Here's how the part is built. I have some questions about the finished solid (model axes, mm). Face numbers are marked on the shaded views. A direction names the side the tool comes from. Round coordinates to 2 decimals unless told otherwise and drop trailing zeros. Order: outer loops, then holes, each group sorted by start corner. A loop starts at its lowest first (then second) coordinate and runs counter-clockwise, first axis right, second up. Notation, with made-up numbers: (64.25, 53.5) -> (75.25, 53.5) arc R37 cw to (75.25, 90.5) -> close; hole circle Ø8 at (88, 12). An arc over 180 degrees is marked (long way). Use a Markdown table: item, result. Add a question column.
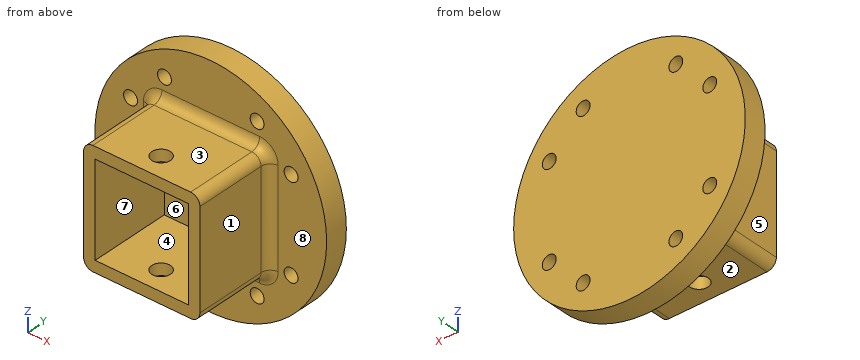
from build123d import *

# Parameters (mm, degrees)
SKETCH2_R               = 31.75
BOSS_EXTRUDE1_DEPTH     = 6.35
SKETCH3_W               = 31.877
SKETCH3_H               = 31.877
BOSS_EXTRUDE2_DEPTH     = 22.225
SKETCH4_W               = 25.527
SKETCH4_H               = 25.527
CUT_EXTRUDE1_DEPTH      = 23.225
SKETCH5_R               = 1.90000001
CUT_EXTRUDE2_DEPTH      = 7.35
SKETCH7_R               = 2.563499953
CUT_EXTRUDE3_DEPTH      = 32.75
CUT_EXTRUDE3_DEPTH_BACK = 32.75
CIRPATTERN2_COUNT       = 4
FILLET2_R               = 2.54
FILLET3_R               = 2.54


with BuildPart() as part:
    # Sketch2 → Boss-Extrude1 (new body)
    with BuildSketch(Plane(origin=(0, 0, 0), x_dir=(1, 0, 0), z_dir=(0, 1, 0))):
        Circle(SKETCH2_R)
    extrude(amount=BOSS_EXTRUDE1_DEPTH)

    # Sketch3 → Boss-Extrude2 (add)
    with BuildSketch(Plane(origin=(0, 0, 0), x_dir=(1, 0, 0), z_dir=(0, 1, 0))):
        Rectangle(SKETCH3_W, SKETCH3_H)
    extrude(amount=-BOSS_EXTRUDE2_DEPTH)

    # Sketch4 → Cut-Extrude1 (cut, through all)
    with BuildSketch(Plane(origin=(0, 0, 0), x_dir=(1, 0, 0), z_dir=(0, 1, 0))):
        Rectangle(SKETCH4_W, SKETCH4_H)
    extrude(amount=-CUT_EXTRUDE1_DEPTH, mode=Mode.SUBTRACT)

    # Sketch5 → Cut-Extrude2 (cut, through all)
    with BuildSketch(Plane(origin=(0, 0, 0), x_dir=(1, 0, 0), z_dir=(0, 1, 0))):
        with Locations((21.997045256, 12.7)):
            Circle(SKETCH5_R)
        with Locations((21.997045256, -12.7)):
            Circle(SKETCH5_R)
    cut_extrude2 = extrude(amount=CUT_EXTRUDE2_DEPTH, mode=Mode.SUBTRACT)

    # Sketch7 → Cut-Extrude3 (cut, two sides)
    with BuildSketch(Plane.XY) as cut_extrude3_sk:
        with Locations((0, -16.002)):
            Circle(SKETCH7_R)
    extrude(amount=CUT_EXTRUDE3_DEPTH, mode=Mode.SUBTRACT)
    extrude(cut_extrude3_sk.sketch, amount=-CUT_EXTRUDE3_DEPTH_BACK, mode=Mode.SUBTRACT)

    # CirPattern2: Cut-Extrude2 ×4 about axis
    cirpattern2_axis = Axis((0, 0, 0), (0, 1, 0))
    for i in range(1, CIRPATTERN2_COUNT):
        add(cut_extrude2.rotate(cirpattern2_axis, i * 360 / CIRPATTERN2_COUNT), mode=Mode.SUBTRACT)

    # Fillet2
    fillet2_edges = [part.edges().sort_by_distance(p)[0] for p in [
        (-15.9385, -11.1125, -15.9385),
        (15.9385, -11.1125, -15.9385),
        (15.9385, -11.1125, 15.9385),
        (-15.9385, -11.1125, 15.9385),
    ]]
    fillet(fillet2_edges, radius=FILLET2_R)

    # Fillet3
    fillet3_edges = [part.edges().sort_by_distance(p)[0] for p in [
        (-15.9385, 0, 0),
        (0, 0, 15.9385),
        (15.9385, 0, 0),
        (0, 0, -15.9385),
        (-15.194551224, 0, 15.194551224),
        (15.194551224, 0, 15.194551224),
        (15.194551224, 0, -15.194551224),
        (-15.194551224, 0, -15.194551224),
    ]]
    fillet(fillet3_edges, radius=FILLET3_R)


solid = part.part
(1) I'm going to push flat-ended pins straight in: P1, Ø2.5, axis at x = 12.7, z = -22, coming from the +Y side; P2, Ø15.5, axis at x = 4, y = -12.5, coming from the -Z side; P3, Ø6.5, axis at y = -5.5, z = -5, coming from the +X side; P4, Ø4.5, axis at x = 22, z = -12.7, coming from the +Y side. Where does each tip first touch, or does it pass through?
(2) If we mould it in two halves opening along X, with no side actions, what happens to the marked faces 5, 6, 7 and 8? For each: pulls with the +X half, pulls with the -X half, needs draft (parallel to the pull), parting line crosses it, or undercut.
(3) I want a section at A-A on y = -19.5. List the corners of the cut face in (x, z) for me, and give its area (3 significant figures).
(4) On a 3-axis mill with a long thin cutter (end or side, diameter ignored), from which of +Z, -Z, +X, -X, +Y, -Y can I reach the whole of each face in a straight line? I mean the marked faces 1, 2, 3 and 4. Say none if no direction works.
(5) I want a section at D-D on y = 1.5. State how many separate pieces and enclosed holes the cut face has, and give its area (3 significant figures).
(6) I want a section at B-B on x = -22.5. List the corners of the cut face in (y, z) for me, and give its area (3 significant figures).
(7) Please list where these lines run through material, in increasing order: probe 1 along X at (y, z) = (-2.5, 4); probe 2 along X at (y, z) = (4.25, 12.7); probe 3 along Y at (x, z) = (-3, -3). Write a range as from..to.
Output:
| question | item | result |
|---|---|---|
| 1 | P1 | through |
| 1 | P2 | z = -15.94 |
| 1 | P3 | x = 15.96 |
| 1 | P4 | y = 6.35 |
| 2 | face 5 | pulls with the -X half |
| 2 | face 6 | undercut |
| 2 | face 7 | undercut |
| 2 | face 8 | needs draft |
| 3 | outline | (-15.94, -13.4) arc R2.54 ccw to (-13.4, -15.94) -> (13.4, -15.94) arc R2.54 ccw to (15.94, -13.4) -> (15.94, 13.4) arc R2.54 ccw to (13.4, 15.94) -> (-13.4, 15.94) arc R2.54 ccw to (-15.94, 13.4) -> close; hole (-12.76, -12.76) -> (12.76, -12.76) -> (12.76, 12.76) -> (-12.76, 12.76) -> close |
| 3 | area | 359 mm² |
| 4 | face 1 | +Z, -Z, +X, -Y |
| 4 | face 2 | -Z, +X, -X, -Y |
| 4 | face 3 | +Z, +X, -X, -Y |
| 4 | face 4 | -Y |
| 5 | separate pieces | 1 |
| 5 | enclosed holes | 8 |
| 5 | area | 3,080 mm² |
| 6 | outline | (0, -22.4) -> (6.35, -22.4) -> (6.35, -14.53) -> (0, -14.53) -> close; (0, -10.87) -> (6.35, -10.87) -> (6.35, 10.87) -> (0, 10.87) -> close; (0, 14.53) -> (6.35, 14.53) -> (6.35, 22.4) -> (0, 22.4) -> close |
| 6 | area | 238 mm² |
| 7 | probe 1 | -15.94..-12.76, 12.76..15.94 |
| 7 | probe 2 | -29.1..-23.9, -20.1..20.1, 23.9..29.1 |
| 7 | probe 3 | 0..6.35 |
